The model under review builds one solid part; all positions refer to its coordinate system, in mm. A direction names the side the tool comes from. Coordinates: 2 decimals unless noted, no trailing zeros. Loops run counter-clockwise (first coordinate to the right, second up) from the corner with the lowest first, then second, coordinate; pieces in that order, holes last. Notation, with made-up numbers: (-27.75, -27.75) - (-21.75, -27.75) arc R19 ccw to (-21.75, 9.25) - close; hole circle Ø5 at (74, -30). An arc over 180 degrees is marked (long way). One line per item, written item: value. Start each with the question number.
1. We need section C-C, the plane x = 45. Give the boundary of the cut face in (y, z).
2. To check wall thickness, follow line 1 (X direction, y = 30, z = 14); line 2 (Y direction, x = 45.5, z = 15); line 3 (Y direction, x = 44.5, z = 4.5). State the ranges of each line that lie inside material, in increasing order.
3. We need section B-B, the plane y = 31. Give the boundary of the cut face in (x, z), then the cut area to 3 significant figures.
4. Mouldability with a two-part tool opening along X and no side actions: class faces 3 (the face through (46.849, 37, 18)), 4 (the face through (48, 38.265, 18)), 5 (the face through (49.849, 33, 18)), 6 (the face through (45.18, 34.69, 17.99)) as +X half, -X half, draft (parallel to the pull), parting line (faces both ways), or undercut.
5. We need section A-A, the plane z = 36. Give the boundary of the cut face in (x, y).
6. Insertion check: P1, Ø3, axis at x = 44.5, z = 16.5, coming from the +Y side; P2, Ø1, axis at x = 45.5, z = 0.5, coming from the -Y side; P3, Ø5, axis at y = 31.5, z = 35.5, coming from the -X side. Each pin has a flat end and moves straight along its axis. Give the tip position at first contact, or say it passes through.
7. For faces 1 (the face through (43.549, 36, 18)), 2 (the face through (45.22, 36.73, 17.99)), list the 3-axis set-ups (+Z, -Z, +X, -X, +Y, -Y) from which the entire face can be reached by the end or side of a thin tool; tool diameter is ignored.
Autodesk Inventor part; units mm, degrees
ref_plane "Work Plane2" through (46.8486, 38.2651, 40.1765) normal (0, 0, 1) x (0, 1, 0)
ref_plane "YZ Plane" through (0, 0, 0) normal (1, 0, 0) x (0, 1, 0)
ref_plane "XZ Plane" through (0, 0, 0) normal (0, 1, 0) x (-1, 0, 0)
ref_plane "Work Plane2" through (46.8486, 38.2651, 40.1765) normal (0, 0, 1) x (0, 1, 0)
sketch "Sketch2" plane through (46.8486, 38.2651, 40.1765) normal (0, 0, 1) x (0, 1, 0)
  line L0 (-3.3829, 0) -> (-4, 3.5)
  line L1 (-1.6171, 0) -> (-3.3829, 0)
  line L2 (-1, 3.5) -> (-1.6171, 0)
  line L3 (-4, 3.5) -> (-1, 3.5)
  line L4 (-3.8632, 3.3) -> (-3.2813, 0)
  line L5 (-1.8202, 0) -> (-1.2384, 3.3)
  line L6 (-1.2384, 3.3) -> (-3.8632, 3.3)
  line L7 (-1.8202, 0) -> (-1.6171, 0)
  line L8 (0, 0) -> (0, -3)
  line L9 (-3.2813, 0) -> (-3.3829, 0)
  line L10 (-3.3829, 0) -> (-4, 3.5)
  line L11 (-4, 3.5) -> (-1, 3.5)
  line L12 (-1, 3.5) -> (-1.6171, 0)
  line L13 (0, 0) -> (-1.6171, 0)
  line L14 (0, 15) -> (0, 0)
  line L15 (0, 15) -> (-5, 15)
  line L16 (-5, 0) -> (-5, 15)
  line L17 (-3.3829, 0) -> (-5, 0)
  line L18 (-5, 0) -> (-5, -3)
  line L19 (-5, -3) -> (0, -3)
  line L20 (0, 0) -> (-1.8202, 0)
  line L21 (-3.2813, 0) -> (-5, 0)
  point P0 (-38.2651, 46.8486)
  dimension "d0" = 0.1
  dimension "d1" = 0.2
  dimension "d2" = 3
  dimension "d9" = 90
extrude "Extrusion1" add sketch "Sketch2" against normal blind 45 contours L1 L13 L8 L19 L18 L17 | L4 L6 L5 L1
sketch "Sketch6" plane through (46.8486, 33.2651, 40.1765) normal (0, -1, 0) x (1, 0, 0)
  line L0 (0, 0) -> (0, -45)
  line L1 (0, -45) -> (3, -45)
  line L2 (0, 0) -> (3, 0)
  line L3 (3, 0) -> (3, -45)
  line L4 (3, -45) -> (0, -45)
  line L5 (0, -45) -> (0, 0)
  point P0 (-46.8486, -40.1765)
extrude "Extrusion2" add sketch "Sketch6" along normal blind 5
properties part number "Rack Gripper"
Findings below:
1. outline: (34.66, -4.82) - (36.77, -4.82) - (36.77, 40.18) - (34.66, 40.18) - close
2. line 1: 46.85 to 49.85
2. line 2: 34.75 to 36.68
2. line 3: 34.57 to 36.86
3. outline: (46.85, -4.82) - (49.85, -4.82) - (49.85, 40.18) - (46.85, 40.18) - close
3. area: 135 mm2
4. face 3: undercut
4. face 4: draft
4. face 5: +X half
4. face 6: undercut
5. outline: (43.55, 34.4) - (46.85, 34.98) - (46.85, 28.27) - (49.85, 28.27) - (49.85, 38.27) - (46.85, 38.27) - (46.85, 36.44) - (43.55, 37.03) - close
6. P1: y = 37.03
6. P2: y = 34.66
6. P3: x = 46.85
7. face 1: +Z, -Z, -X, +Y, -Y
7. face 2: +Z, -Z, +Y
